The model under review builds one solid part; all positions refer to its coordinate system, in mm. A direction names the side the tool comes from. Round coordinates to 2 decimals unless told otherwise and drop trailing zeros. Order: outer loops, then holes, each group sorted by start corner. A loop starts at its lowest first (then second) coordinate and runs counter-clockwise, first axis right, second up. Notation, with made-up numbers: (19.25, 16.25) - (53.25, 16.25) arc R9 cw to (53.25, 25.25) - close; hole circle Ø9 at (32, -5.5). An arc over 180 degrees is marked (long way). One line per question, with ' | ' between items. Start each with the question number.
Item 1: For L1, parallel to X at y = 1.45, z = -10; L2, parallel to X at y = -80.5, z = 1.7; L3, parallel to Y at x = 63.5, z = 1.75, list the stretches that pass through material, from the lowest coordinate up. Write a range as [from, to].
Item 2: Add section B-B on y = -54. State the section outline as (x, z) points, and give its area (3 significant figures).
Item 3: Draft analysis for pull direction X (two halves, no side actions). For faces 1 (the face through (-38.07, -87.15, 1.48)), 2 (the face through (199.145, -49.317, 1.479)), 3 (the face through (81, -44, 0)), 4 (the face through (108.46, -25.87, 1.52)), state which applies: +X half, -X half, draft (parallel to the pull), parting line (faces both ways), or undercut.
Item 4: Tool access review of faces 5 (the face through (24, 0, -6)), 6 (the face through (143.5, -5.7, 0.4)), 7 (the face through (81, -44, 3)), 8 (the face through (0, -13.6, 0.4)), 9 (the face through (175.189, -73.814, 1.479)): name each direction out of +Z, -Z, +X, -X, +Y, -Y from which nothing blocks a thin tool from reaching the whole face with its end or side.
Item 5: Insertion check: pin 1 Ø4.5 at (x, z) = (104.4, -10) entering from -Y; pin 2 Ø1.5 at (y, z) = (1.5, -8.5) entering from -X; pin 3 Ø0.9 at (x, z) = (72.5, 1.5) entering from +Y. Each pin has a flat end and moves straight along its axis. Give the tip position at first contact, or say it passes through.
Item 6: Add section A-A on y = -8. State the section outline as (x, z) points, and give its area (4 significant figures).
from build123d import *

# Parameters (mm, degrees)
BOSS_EXTRUDE1_DEPTH = 3
SKETCH2_R           = 1.9
SKETCH2_R_2         = 6.25
CUT_EXTRUDE1_DEPTH  = 4
BOSS_EXTRUDE2_DEPTH = 143.5
SKETCH4_W           = 47
SKETCH4_H           = 16
CUT_EXTRUDE2_DEPTH  = 3
SKETCH5_R           = 1.9
CUT_EXTRUDE3_DEPTH  = 94


with BuildPart() as part:
    # Sketch1 → Boss-Extrude1 (new body)
    with BuildSketch(Plane.XY):
        with BuildLine():
            Line((0, 0), (143.5, 0))
            Line((143.5, 0), (143.5, -25))
            ThreePointArc((143.5, -25), (145.839555569, -31.427876097), (151.763518223, -34.84807753))
            Line((151.763518223, -34.84807753), (191.155828344, -41.794004637))
            ThreePointArc((191.155828344, -41.794004637), (199.182306638, -49.477686028), (195.155110931, -59.83360261))
            Line((195.155110931, -59.83360261), (154.655807102, -88.191520443))
            ThreePointArc((154.655807102, -88.191520443), (151.927100734, -89.537169507), (148.920042738, -90))
            Line((148.920042738, -90), (-31.079957262, -90))
            ThreePointArc((-31.079957262, -90), (-38.151025073, -87.071067812), (-41.079957262, -80))
            Line((-41.079957262, -80), (-41.079957262, -70))
            ThreePointArc((-41.079957262, -70), (-39.51387172, -64.627003917), (-35.306139879, -60.93692213))
            Line((-35.306139879, -60.93692213), (-4.054276098, -46.363938717))
            ThreePointArc((-4.054276098, -46.363938717), (-1.099678559, -43.772826218), (0, -40))
            Line((0, -40), (0, 0))
        make_face()
    extrude(amount=BOSS_EXTRUDE1_DEPTH)

    # Sketch2 → Cut-Extrude1 (cut, through all)
    with BuildSketch(Plane.XY.offset(3)):
        with Locations((188.758637025, -47.565112823)):
            Circle(SKETCH2_R)
        with Locations((135.640436691, -80.5)):
            Circle(SKETCH2_R)
        with Locations((79.840436691, -80.5)):
            Circle(SKETCH2_R)
        with Locations((24.640436691, -80.5)):
            Circle(SKETCH2_R)
        with Locations((102.5, -27.75)):
            Circle(SKETCH2_R_2)
        with Locations((136.140436691, -22)):
            Circle(SKETCH2_R)
        with BuildLine():
            Line((-28.634563309, -82.4), (-34.084563309, -82.4))
            ThreePointArc((-34.084563309, -82.4), (-35.984563309, -80.5), (-34.084563309, -78.6))
            Line((-34.084563309, -78.6), (-28.634563309, -78.6))
            ThreePointArc((-28.634563309, -78.6), (-26.734563309, -80.5), (-28.634563309, -82.4))
        make_face()
    extrude(amount=-CUT_EXTRUDE1_DEPTH, mode=Mode.SUBTRACT)

    # Sketch3 → Boss-Extrude2 (add)
    with BuildSketch(Plane(origin=(143.5, 0, 0), x_dir=(0, 0, -1), z_dir=(1, 0, 0))):
        with BuildLine():
            Line((0, 0), (13, 0))
            Line((13, 0), (13, 3))
            Line((13, 3), (0, 3))
            ThreePointArc((0, 3), (-2.121320344, 2.121320344), (-3, 0))
            Line((-3, 0), (0, 0))
        make_face()
    extrude(amount=-BOSS_EXTRUDE2_DEPTH)

    # Sketch4 → Cut-Extrude2 (cut)
    with BuildSketch(Plane(origin=(0, 3, 0), x_dir=(1, 0, 0), z_dir=(0, 1, 0))):
        with Locations((71, 5)):
            Rectangle(SKETCH4_W, SKETCH4_H)
    extrude(amount=-CUT_EXTRUDE2_DEPTH, mode=Mode.SUBTRACT)

    # Sketch5 → Cut-Extrude3 (cut, through all)
    with BuildSketch(Plane(origin=(0, 3, 0), x_dir=(1, 0, 0), z_dir=(0, 1, 0))):
        with Locations((8.4, 10)):
            Circle(SKETCH5_R)
        with Locations((37.6, 10)):
            Circle(SKETCH5_R)
        with Locations((104.4, 10)):
            Circle(SKETCH5_R)
        with Locations((133.6, 10)):
            Circle(SKETCH5_R)
    extrude(amount=-CUT_EXTRUDE3_DEPTH, mode=Mode.SUBTRACT)


solid = part.part
Determined:
1) L1: [0, 6.5], [10.3, 35.7], [39.5, 47.5], [94.5, 102.5], [106.3, 131.7], [135.5, 143.5] | L2: [-41.07, -35.98], [-26.73, 22.74], [26.54, 77.94], [81.74, 133.74], [137.54, 165.64] | L3: [-90, 0]
2) outline: (-20.43, 0) - (199.14, 0) - (199.14, 3) - (-20.43, 3) - close | area: 659 mm2
3) face 1: -X half | face 2: +X half | face 3: draft | face 4: undercut
4) face 5: -Z, +X, -X, -Y | face 6: +Z, -Z, +X, +Y | face 7: +Z, +X, -X, +Y, -Y | face 8: +Z, -Z, -X, +Y | face 9: +Z, -Z, +X, -Y
5) pin 1: y = 0 | pin 2: x = 0 | pin 3: y = 0
6) outline: (0, 0) - (143.5, 0) - (143.5, 3) - (0, 3) - close | area: 430.5 mm2
